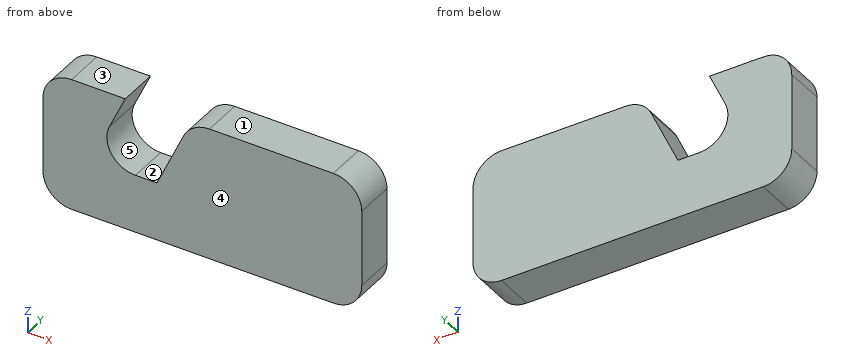
from build123d import *

# Parameters (mm, degrees)
F1_DEPTH = 7
F2_R     = 5


with BuildPart() as f1:
    # F0 (on Front) → F1 (new body)
    with BuildSketch(Plane.XZ):
        Polygon((0, 23.336001), (0, 0), (55.836968, 0), (55.836968, 23.336001), (25.954563, 23.336001), (19.947276, 10.243195), (8.394799, 10.243195), (14.402086, 23.336001), align=None)
    extrude(amount=F1_DEPTH)

    # F2
    f2_edges = [f1.edges().sort_by_distance(p)[0] for p in [
        (55.836968, -3.5, 23.336001),
        (55.836968, -3.5, 0),
        (25.954563, -3.5, 23.336001),
        (0, -3.5, 0),
        (8.394799, -3.5, 10.243195),
        (0, -3.5, 23.336001),
    ]]
    fillet(f2_edges, radius=F2_R)


solid = f1.part
Can you work these out from the model? Positions are in its coordinate system, mm. Face numbers are marked on the shaded views. A direction names the side the tool comes from. Coordinates: 2 decimals unless noted, no trailing zeros. Write each loop counter-clockwise with the first axis right and the second up, starting at its lowest first coordinate (ties: lowest second). Pieces come first, ordered by that corner, then holes. Notation, with made-up numbers: (32.25, 26) -> (82.25, 26) arc R23 ccw to (82.25, 51) -> close; hole circle Ø8 at (66.5, 18.25). An arc over 180 degrees is marked (long way). Write each question's results on one line, items separated by ' | '. Start each with the question number.
Item 1: If we section it at A-A, the plane z = 14.25: Write out the boundary of the cut face in (x, y).
Item 2: If we section it at D-D, the plane z = 21.25: Write out the boundary of the cut face in (x, y).
Item 3: Thinking about a two-plate mould opening in Z: for the marked faces 3, 4 and 5, which applies, released by +Z, released by -Z, zero draft, split by the parting line, or undercut?
Item 4: Please list where these lines run through material, in increasing order: probe 1 along Z at (x, y) = (18, -1.5); probe 2 along Z at (x, y) = (51, -6.25); probe 3 along X at (y, z) = (-3, 17.25).
Item 5: If we section it at B-B, the plane y = -5.75: Write out the boundary of the cut face in (x, z), and give its area (3 significant figures).
Item 6: If we section it at C-C, the plane x = 17: Write out the boundary of the cut face in (y, z), and give its area (3 significant figures).
Item 7: I'm going to push flat-ended pins straight in: P1, Ø2, axis at y = -4, z = 3, coming from the -X side; P2, Ø1.1, axis at x = 17.5, y = -4.5, coming from the +Z side. Where does each tip first touch, or does it pass through?
Item 8: On a 3-axis mill with a long thin cutter (end or side, diameter ignored), from which of +Z, -Z, +X, -X, +Y, -Y can I reach the whole of each face in a straight line? I mean the marked faces 1 and 2. Say none if no direction works.
Answer block:
1) outline: (0, -7) -> (11.29, -7) -> (11.29, 0) -> (0, 0) -> close; (21.79, -7) -> (55.84, -7) -> (55.84, 0) -> (21.79, 0) -> close
2) outline: (0.94, -7) -> (13.44, -7) -> (13.44, 0) -> (0.94, 0) -> close; (25.1, -7) -> (54.9, -7) -> (54.9, 0) -> (25.1, 0) -> close
3) face 3: released by +Z | face 4: zero draft | face 5: undercut
4) probe 1: 0 to 10.24 | probe 2: 0 to 23.33 | probe 3: 0 to 11.61, 23.16 to 55.84
5) outline: (0, 5) arc R5 ccw to (5, 0) -> (50.84, 0) arc R5 ccw to (55.84, 5) -> (55.84, 18.34) arc R5 ccw to (50.84, 23.34) -> (29.16, 23.34) arc R5 ccw to (24.62, 20.42) -> (19.95, 10.24) -> (16.19, 10.24) arc R5 cw to (11.65, 17.33) -> (14.4, 23.34) -> (5, 23.34) arc R5 ccw to (0, 18.34) -> close | area: 1,140 mm²
6) outline: (-7, 0) -> (0, 0) -> (0, 10.24) -> (-7, 10.24) -> close | area: 71.7 mm²
7) P1: x = 0.1 | P2: z = 10.24
8) face 1: +Z, +X, -X, +Y, -Y | face 2: +Z, +Y, -Y
